Design review of the part built by this model. Coordinates are the model's own, in mm. A direction names the side the tool comes from. Coordinates: 2 decimals unless noted, no trailing zeros. Write each loop counter-clockwise with the first axis right and the second up, starting at its lowest first coordinate (ties: lowest second). Pieces come first, ordered by that corner, then holes. Notation, with made-up numbers: (9, 84) - (22, 84) arc R18 cw to (22, 90) - close; hole circle Ø10 at (42.5, -35). An arc over 180 degrees is marked (long way). Answer as CSV lines item,"result". Start each with the question number.
Q1. Machinability: for faces 1 (the face through (-17.968, 0.843, 1.479)), 2 (the face through (-1, 3.75, 1)), 3 (the face through (-1, -11, 0)), which of the approach directions +Z, -Z, +X, -X, +Y, -Y give a long, thin tool a straight path to every point of the face, cutting with its end or side? Answer none if there is none.
Q2. We need section C-C (x = -20). Write out the cut boundary in (y, z).
Q3. We need section B-B (x = 1.5). Write out the cut boundary in (y, z), plus the area to 4 significant figures.
Q4. We need section A-A (y = 0). Write out the cut boundary in (x, z), plus the area to 3 significant figures.
Q5. For line 1 along X through (y, z) = (0, 2.35); line 2 along Y through (x, z) = (20, 1.8); line 3 along Z through (x, y) = (18.5, -5), list the stretches that pass through material, from the lowest coordinate up. Write a range as [from, to].
Q6. We need section D-D (y = 5.5). Write out the cut boundary in (x, z), plus the area to 3 significant figures.
Q7. Mouldability with a two-part tool opening along Y and no side actions: class faces 4 (the face through (20, 0, 0)), 5 (the face through (-1, -19, -2)), 6 (the face through (-20, 0, 0)), 7 (the face through (-1, 0, -5)) as pulls with the +Y half, pulls with the -Y half, needs draft (parallel to the pull), parting line crosses it, or undercut.
Q8. Clearance check with flat-ended pins moving along their axes: pin 1 (17 mm diameter, centred on x = -5.5, y = -9.5, fed in from +Z); pin 2 (3.5 mm diameter, centred on x = -19, z = 2, fed in from +Y); pin 3 (6 mm diameter, centred on x = 22, y = -7, fed in from +Z). State where each tip first meets the part, or that it passes through.
from build123d import *

# Parameters (mm, degrees)
F0_W     = 80
F0_H     = 15.25
F0_H_2   = 7.5
F1_DEPTH = 5
F2_DEPTH = 3
F4_D     = 4.4
F4_DEPTH = 3.001


with BuildPart() as f1:
    # F0 (on Top) → F1 (new body)
    with BuildSketch(Plane.XY):
        with Locations((0, 11.375)):
            Rectangle(F0_W, F0_H)
        with Locations((0, -11.375)):
            Rectangle(F0_W, F0_H)
        Rectangle(F0_W, F0_H_2)
    extrude(amount=-F1_DEPTH)

    # F0 (on Top) → F2 (join)
    with BuildSketch(Plane.XY):
        Rectangle(F0_W, F0_H_2)
    extrude(amount=F2_DEPTH)

    # F4 (through all, one way)
    with BuildSketch(Plane(origin=(0, 0, 0), x_dir=(1, 0, 0), z_dir=(0, 0, -1))):
        with Locations((-20, 0), (20, 0)):
            Circle(F4_D / 2)
    extrude(amount=-F4_DEPTH, mode=Mode.SUBTRACT)


solid = f1.part
Results list:
1,face 1,"+Z"
1,face 2,"+Z, +X, -X, +Y"
1,face 3,"+Z, +X, -X, -Y"
2,outline,"(-19, -5) - (19, -5) - (19, 0) - (3.75, 0) - (3.75, 3) - (2.2, 3) - (2.2, 0) - (-2.2, 0) - (-2.2, 3) - (-3.75, 3) - (-3.75, 0) - (-19, 0) - close"
3,outline,"(-19, -5) - (19, -5) - (19, 0) - (3.75, 0) - (3.75, 3) - (-3.75, 3) - (-3.75, 0) - (-19, 0) - close"
3,area,"212.5 mm2"
4,outline,"(-40, -5) - (40, -5) - (40, 3) - (22.2, 3) - (22.2, 0) - (17.8, 0) - (17.8, 3) - (-17.8, 3) - (-17.8, 0) - (-22.2, 0) - (-22.2, 3) - (-40, 3) - close"
4,area,"614 mm2"
5,line 1,"x = [-40, -22.2], [-17.8, 17.8], [22.2, 40]"
5,line 2,"y = [-3.75, -2.2], [2.2, 3.75]"
5,line 3,"z = [-5, 0]"
6,outline,"(-40, -5) - (40, -5) - (40, 0) - (-40, 0) - close"
6,area,"400 mm2"
7,face 4,"undercut"
7,face 5,"pulls with the -Y half"
7,face 6,"undercut"
7,face 7,"needs draft"
8,pin 1,"stops at z = 3"
8,pin 2,"stops at y = 3.75"
8,pin 3,"stops at z = 0"
